Work out the finished part from the listing and answer in its coordinate system (mm). Face numbers are marked on the shaded views. A direction names the side the tool comes from. Round coordinates to 2 decimals unless told otherwise and drop trailing zeros. Write each loop counter-clockwise with the first axis right and the second up, starting at its lowest first coordinate (ties: lowest second). Pieces come first, ordered by that corner, then holes.
1. Find section A-A (z = -1). Write down the section's boundary in (x, y).
2. Find section D-D (z = -20). Write down the section's boundary in (x, y).
3. Straight lines are drawn through the part: probe 1 along Y at (x, z) = (0, 2.1); probe 2 along X at (y, z) = (0, -19.3); probe 3 along X at (y, z) = (0, -3.65). For each, find the intervals that lie inside material, in ascending order.
4. Find section B-B (y = 19). Write down the section's boundary in (x, z), and give its area (3 significant figures).
5. Determine the mould class of the marked faces 1, 2, 3 and 4 for opening direction X: pulls with the +X half, pulls with the -X half, needs draft (parallel to the pull), parting line crosses it, or undercut.
6. Find section C-C (x = -21.5). Write down the section's boundary in (y, z), and give its area (3 significant figures).
7. Flat-ended cylindrical pins translate along their axes: pin 1 Ø17.5 at (x, y) = (0.5, 0.5) entering from +Z; pin 2 Ø5 at (y, z) = (-1.5, -24) entering from +X; pin 3 Ø1.4 at (x, y) = (-10, 10) entering from +Z; pin 4 Ø5 at (x, z) = (-12, -2) entering from -Y. Find the tip coordinate at first contact, or state that the pin passes through.
8. A tool of negligible diameter and unlimited length cuts with its end or side. For the marked faces 5, 6 and 7, from which of +Z, -Z, +X, -X, +Y, -Y can it reach the whole face along a straight path? Write none if from no direction.
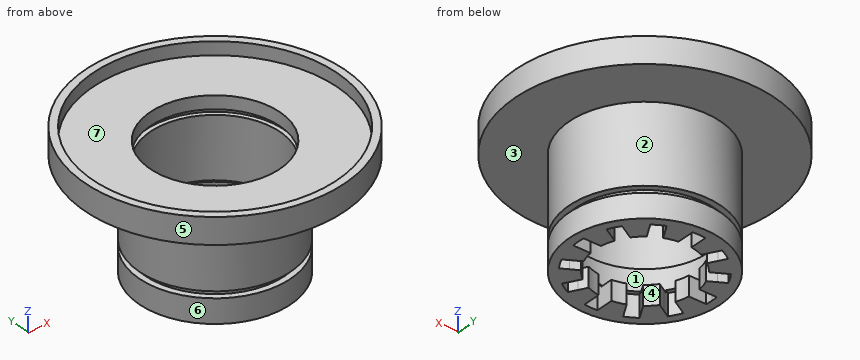
```python
from build123d import *

# Parameters (mm, degrees)
SKETCH_1_R          = 30
SKETCH_1_R_2        = 28.251
EXTRUDE_1_DEPTH     = 3
SKETCH_2_R          = 30
SKETCH_2_R_2        = 15
EXTRUDE_2_DEPTH     = 3
SKETCH_4_R          = 17.5
SKETCH_4_R_2        = 15
EXTRUDE_3_DEPTH     = 20
SKETCH_5_R          = 17.5
SKETCH_5_R_2        = 14.5
EXTRUDE_4_DEPTH     = 0.5
SKETCH_6_W          = 1.5
SKETCH_6_H          = 1.4
SKETCH_7_W          = 1.2
SKETCH_7_H          = 1.05
SKETCH_8_R          = 15
SKETCH_8_R_2        = 14.5
EXTRUDE_5_DEPTH     = 4.8
SKETCH_9_R          = 17.5
SKETCH_9_R_2        = 11.5
EXTRUDE_6_DEPTH     = 4.5
CUT_EXTRUDE_1_DEPTH = 5


with BuildPart() as part:
    # 草图1 → 凸台-拉伸1 (new body)
    with BuildSketch(Plane.XY):
        Circle(SKETCH_1_R)
        Circle(SKETCH_1_R_2, mode=Mode.SUBTRACT)
    extrude(amount=EXTRUDE_1_DEPTH)

    # 草图2 → 凸台-拉伸2 (add)
    with BuildSketch(Plane.XY):
        Circle(SKETCH_2_R)
        Circle(SKETCH_2_R_2, mode=Mode.SUBTRACT)
    extrude(amount=-EXTRUDE_2_DEPTH)

    # 草图4 → 凸台-拉伸3 (add)
    with BuildSketch(Plane(origin=(0, 0, -3), x_dir=(-1, 0, 0), z_dir=(0, 0, -1))):
        Circle(SKETCH_4_R)
        Circle(SKETCH_4_R_2, mode=Mode.SUBTRACT)
    extrude(amount=EXTRUDE_3_DEPTH)

    # 草图5 → 凸台-拉伸4 (add)
    with BuildSketch(Plane(origin=(0, 0, -23), x_dir=(-1, 0, 0), z_dir=(0, 0, -1))):
        Circle(SKETCH_5_R)
        Circle(SKETCH_5_R_2, mode=Mode.SUBTRACT)
    extrude(amount=EXTRUDE_4_DEPTH)

    # 草图6 → 切除-旋转1 (revolve, cut)
    with BuildSketch(Plane(origin=(0, 0, 0), x_dir=(0, 0, -1), z_dir=(1, 0, 0))):
        with Locations((21.75, 16.8)):
            Rectangle(SKETCH_6_W, SKETCH_6_H)
    revolve(axis=Axis((0, 0, 3), (0, 0, -1)), mode=Mode.SUBTRACT)

    # 草图7 → 切除-旋转2 (revolve, cut)
    with BuildSketch(Plane(origin=(0, 0, 0), x_dir=(0, 0, -1), z_dir=(1, 0, 0))):
        with Locations((3.6, 15.498648932)):
            Rectangle(SKETCH_7_W, SKETCH_7_H)
    revolve(axis=Axis((0, 0, 3), (0, 0, -1)), mode=Mode.SUBTRACT)

    # 草图8 → 凸台-拉伸5 (add)
    with BuildSketch(Plane(origin=(0, 0, -23), x_dir=(-1, 0, 0), z_dir=(0, 0, -1))):
        Circle(SKETCH_8_R)
        Circle(SKETCH_8_R_2, mode=Mode.SUBTRACT)
    extrude(amount=-EXTRUDE_5_DEPTH)

    # 草图9 → 凸台-拉伸6 (add)
    with BuildSketch(Plane(origin=(0, 0, -23.5), x_dir=(-1, 0, 0), z_dir=(0, 0, -1))):
        Circle(SKETCH_9_R)
        Circle(SKETCH_9_R_2, mode=Mode.SUBTRACT)
    extrude(amount=EXTRUDE_6_DEPTH)

    # 草图10 → 切除-拉伸1 (cut)
    with BuildSketch(Plane(origin=(0, 0, -28), x_dir=(-1, 0, 0), z_dir=(0, 0, -1))):
        with BuildLine():
            ThreePointArc((-1.5, 11.401754251), (0, 11.5), (1.5, 11.401754251))
            Line((1.5, 11.401754251), (1.5, 13.5))
            Line((1.5, 13.5), (1.5, 15.427248621))
            ThreePointArc((1.5, 15.427248621), (0, 15.5), (-1.5, 15.427248621))
            Line((-1.5, 15.427248621), (-1.5, 13.5))
            Line((-1.5, 13.5), (-1.5, 11.401754251))
        make_face()
        with BuildLine():
            Line((6.414586205, 14.110389216), (5.450961894, 12.441342951))
            Line((5.450961894, 12.441342951), (4.40183902, 10.624208829))
            ThreePointArc((4.40183902, 10.624208829), (5.75, 9.959292144), (6.999915231, 9.124208829))
            Line((6.999915231, 9.124208829), (8.049038106, 10.941342951))
            Line((8.049038106, 10.941342951), (9.012662416, 12.610389216))
            ThreePointArc((9.012662416, 12.610389216), (7.75, 13.423393759), (6.414586205, 14.110389216))
        make_face()
        with BuildLine():
            Line((10.941342951, 8.049038106), (9.124208829, 6.999915231))
            ThreePointArc((9.124208829, 6.999915231), (9.959292144, 5.75), (10.624208829, 4.40183902))
            Line((10.624208829, 4.40183902), (12.441342951, 5.450961894))
            Line((12.441342951, 5.450961894), (14.110389216, 6.414586205))
            ThreePointArc((14.110389216, 6.414586205), (13.423393759, 7.75), (12.610389216, 9.012662416))
            Line((12.610389216, 9.012662416), (10.941342951, 8.049038106))
        make_face()
        with BuildLine():
            Line((13.5, 1.5), (11.401754251, 1.5))
            ThreePointArc((11.401754251, 1.5), (11.475412278, 0.751606983), (11.5, 0))
            ThreePointArc((11.5, 0), (11.475412278, -0.751606983), (11.401754251, -1.5))
            Line((11.401754251, -1.5), (13.5, -1.5))
            Line((13.5, -1.5), (15.427248621, -1.5))
            ThreePointArc((15.427248621, -1.5), (15.481801472, -0.750881609), (15.5, 0))
            ThreePointArc((15.5, 0), (15.481801472, 0.750881609), (15.427248621, 1.5))
            Line((15.427248621, 1.5), (13.5, 1.5))
        make_face()
        with BuildLine():
            Line((12.441342951, -5.450961894), (10.624208829, -4.40183902))
            ThreePointArc((10.624208829, -4.40183902), (9.959292144, -5.75), (9.124208829, -6.999915231))
            Line((9.124208829, -6.999915231), (10.941342951, -8.049038106))
            Line((10.941342951, -8.049038106), (12.610389216, -9.012662416))
            ThreePointArc((12.610389216, -9.012662416), (13.423393759, -7.75), (14.110389216, -6.414586205))
            Line((14.110389216, -6.414586205), (12.441342951, -5.450961894))
        make_face()
        with BuildLine():
            Line((8.049038106, -10.941342951), (6.999915231, -9.124208829))
            ThreePointArc((6.999915231, -9.124208829), (5.75, -9.959292144), (4.40183902, -10.624208829))
            Line((4.40183902, -10.624208829), (5.450961894, -12.441342951))
            Line((5.450961894, -12.441342951), (6.414586205, -14.110389216))
            ThreePointArc((6.414586205, -14.110389216), (7.75, -13.423393759), (9.012662416, -12.610389216))
            Line((9.012662416, -12.610389216), (8.049038106, -10.941342951))
        make_face()
        with BuildLine():
            Line((1.5, -13.5), (1.5, -11.401754251))
            ThreePointArc((1.5, -11.401754251), (0, -11.5), (-1.5, -11.401754251))
            Line((-1.5, -11.401754251), (-1.5, -13.5))
            Line((-1.5, -13.5), (-1.5, -15.427248621))
            ThreePointArc((-1.5, -15.427248621), (0, -15.5), (1.5, -15.427248621))
            Line((1.5, -15.427248621), (1.5, -13.5))
        make_face()
        with BuildLine():
            ThreePointArc((-4.40183902, -10.624208829), (-5.75, -9.959292144), (-6.999915231, -9.124208829))
            Line((-6.999915231, -9.124208829), (-8.049038106, -10.941342951))
            Line((-8.049038106, -10.941342951), (-9.012662416, -12.610389216))
            ThreePointArc((-9.012662416, -12.610389216), (-7.75, -13.423393759), (-6.414586205, -14.110389216))
            Line((-6.414586205, -14.110389216), (-5.450961894, -12.441342951))
            Line((-5.450961894, -12.441342951), (-4.40183902, -10.624208829))
        make_face()
        with BuildLine():
            ThreePointArc((-9.124208829, -6.999915231), (-9.959292144, -5.75), (-10.624208829, -4.40183902))
            Line((-10.624208829, -4.40183902), (-12.441342951, -5.450961894))
            Line((-12.441342951, -5.450961894), (-14.110389216, -6.414586205))
            ThreePointArc((-14.110389216, -6.414586205), (-13.423393759, -7.75), (-12.610389216, -9.012662416))
            Line((-12.610389216, -9.012662416), (-10.941342951, -8.049038106))
            Line((-10.941342951, -8.049038106), (-9.124208829, -6.999915231))
        make_face()
        with BuildLine():
            ThreePointArc((-11.401754251, -1.5), (-11.5, 0), (-11.401754251, 1.5))
            Line((-11.401754251, 1.5), (-13.5, 1.5))
            Line((-13.5, 1.5), (-15.427248621, 1.5))
            ThreePointArc((-15.427248621, 1.5), (-15.5, 0), (-15.427248621, -1.5))
            Line((-15.427248621, -1.5), (-13.5, -1.5))
            Line((-13.5, -1.5), (-11.401754251, -1.5))
        make_face()
        with BuildLine():
            ThreePointArc((-10.624208829, 4.40183902), (-9.959292144, 5.75), (-9.124208829, 6.999915231))
            Line((-9.124208829, 6.999915231), (-10.941342951, 8.049038106))
            Line((-10.941342951, 8.049038106), (-12.610389216, 9.012662416))
            ThreePointArc((-12.610389216, 9.012662416), (-13.423393759, 7.75), (-14.110389216, 6.414586205))
            Line((-14.110389216, 6.414586205), (-12.441342951, 5.450961894))
            Line((-12.441342951, 5.450961894), (-10.624208829, 4.40183902))
        make_face()
        with BuildLine():
            ThreePointArc((-6.999915231, 9.124208829), (-5.75, 9.959292144), (-4.40183902, 10.624208829))
            Line((-4.40183902, 10.624208829), (-5.450961894, 12.441342951))
            Line((-5.450961894, 12.441342951), (-6.414586205, 14.110389216))
            ThreePointArc((-6.414586205, 14.110389216), (-7.75, 13.423393759), (-9.012662416, 12.610389216))
            Line((-9.012662416, 12.610389216), (-8.049038106, 10.941342951))
            Line((-8.049038106, 10.941342951), (-6.999915231, 9.124208829))
        make_face()
    extrude(amount=-CUT_EXTRUDE_1_DEPTH, mode=Mode.SUBTRACT)


solid = part.part
```
Worked answers:
1. outline: circle Ø60 at (0, 0); hole circle Ø30 at (0, 0)
2. outline: circle Ø35 at (0, 0); hole circle Ø29 at (0, 0)
3. probe 1: y = -30 to -28.25, 28.25 to 30
3. probe 2: x = -17.5 to -14.5, 14.5 to 17.5
3. probe 3: x = -17.5 to -16.02, 16.02 to 17.5
4. outline: (-23.22, -3) - (23.22, -3) - (23.22, 3) - (20.91, 3) - (20.91, 0) - (-20.91, 0) - (-20.91, 3) - (-23.22, 3) - close
4. area: 153 mm2
5. face 1: undercut
5. face 2: parting line crosses it
5. face 3: needs draft
5. face 4: undercut
6. outline: (-20.92, -3) - (20.92, -3) - (20.92, 3) - (18.33, 3) - (18.33, 0) - (-18.33, 0) - (-18.33, 3) - (-20.92, 3) - close
6. area: 141 mm2
7. pin 1: passes through
7. pin 2: stops at x = 17.5
7. pin 3: stops at z = -18.2
7. pin 4: stops at y = -28.46
8. face 5: +Z, -Z
8. face 6: -Z
8. face 7: +Z
